Autodesk Inventor part; units mm, degrees
ref_plane "YZ Plane" through (0, 0, 0) normal (1, 0, 0) x (0, 1, 0)
ref_plane "XZ Plane" through (0, 0, 0) normal (0, 1, 0) x (-1, 0, 0)
ref_plane "XY Plane" through (0, 0, 0) normal (0, 0, 1) x (1, 0, 0)
sketch "Sketch1" plane through (0, 0, 0) normal (0, 1, 0) x (-1, 0, 0)
  line L0 (87.5, 110) -> (-87.5, 110)
  line L1 (-87.5, 110) -> (-87.5, -110)
  line L2 (-87.5, -110) -> (87.5, -110)
  line L3 (87.5, -110) -> (87.5, 110)
  point P0 (0, 0)
  dimension "d0" = 110
  dimension "d1" = 110
  dimension "d2" = 87.5
  dimension "d3" = 87.5
extrude "Extrusion1" add sketch "Sketch1" along normal blind 4.5
fillet "Fillet1" radius 10 4 edges at (-87.5, 2.25, 110) (-87.5, 2.25, -110) (87.5, 2.25, -110) (87.5, 2.25, 110)
fillet "Fillet2" radius 2 8 edges at (-84.5711, 4.5, 107.0711) (0, 4.5, 110) (84.5711, 4.5, 107.0711) (87.5, 4.5, 0) (84.5711, 4.5, -107.0711) (0, 4.5, -110) (-84.5711, 4.5, -107.0711) (-87.5, 4.5, 0)
sketch "Sketch2" plane through (0, 0, 0) normal (0, -1, 0) x (1, 0, 0)
  circle A0 centre (-80.5, -103) radius 1
  line L0 (77.5, -110) -> (-77.5, -110)
  line L1 (-87.5, -100) -> (-87.5, 100)
  circle A1 centre (79.5, -103) radius 1
  circle A2 centre (-80.5, 102) radius 1
  circle A3 centre (79.5, 102) radius 1
  point P0 (0, 0)
  dimension "d8" = 7
  dimension "d9" = 7
  dimension "d10" = 2
  dimension "d13" = 160
  dimension "d16" = 205
extrude "Extrusion2" add sketch "Sketch2" along normal blind 5
sketch "Sketch4" plane through (0, 4.5, 0) normal (0, 1, 0) x (1, 0, 0)
  line L0 (88.4576, 110.604) -> (88.4576, -111.3884) construction
  line L1 (88.4576, -111.3884) -> (-87.9776, -111.3884) construction
  line L2 (-87.9776, -111.3884) -> (-87.9776, 110.604) construction
  line L3 (-87.9776, 110.604) -> (88.4576, 110.604) construction
  point P0 (0, 0)
decal "Decal1"
decal "Decal2"
decal "Decal3"
decal "Decal4"
decal "Decal5"
decal "Decal6"
decal "Decal7"
decal "Decal8"
decal "Decal9"
properties part number "Solar Panel"
Build history of the part. All positions in model axes, mm. Coordinates: 2 decimals unless noted, no trailing zeros. Order: outer loops, then holes, each group sorted by start corner. A loop starts at its lowest first (then second) coordinate and runs counter-clockwise, first axis right, second up. Notation, with made-up numbers: M 66,-13 L 87,-13 A18 cw 87,-2 Z; hole C -5,-16 d9. An arc over 180 degrees is marked long. One line per question, with ' | ' between items. Start each with the question number.
Q1. Saw through at A-A (x = -40.5). List the corners of the cut face in (y, z), then the cut area to 3 significant figures.
Q2. Saw through at B-B (z = 78.5). List the corners of the cut face in (x, y), then the cut area to 3 significant figures.
Q3. Probe L1, parallel to Y at x = -24, z = 39.5; L2, parallel to X at y = 3.5, z = 32; L3, parallel to Z at x = -46.5, y = 4.25. List the from-to ranges inside material, lowest first. Write a range as from..to.
Q4. Flat gauge pin, fed straight in: pin 1 Ø6 at (x, z) = (-35.5, 28.5) entering from -Y. Where does the tip first touch, or does it go through?
Check values:
1) outline: M 0,-110 L 2.5,-110 A2 ccw 4.5,-108 L 4.5,108 A2 ccw 2.5,110 L 0,110 Z | area: 988 mm2
2) outline: M -87.5,0 L 87.5,0 L 87.5,2.5 A2 ccw 85.5,4.5 L -85.5,4.5 A2 ccw -87.5,2.5 Z | area: 786 mm2
3) L1: y = 0..4.5 | L2: x = -87.23..87.23 | L3: z = -108.97..108.97
4) pin 1: stops at y = 0
